Geometry check sheet. Reference: the model listing, model coordinates, mm. Round coordinates to 2 decimals unless told otherwise and drop trailing zeros. Loops run counter-clockwise (first coordinate to the right, second up) from the corner with the lowest first, then second, coordinate; pieces in that order, holes last. Notation, with made-up numbers: (-38, 54) - (-31, 54) arc R27 ccw to (-31, 93) - close; hole circle Ø3 at (50.5, 62). An arc over 180 degrees is marked (long way). Answer in a Markdown table with one row per item. Add a question column.
Autodesk Inventor part; units mm, degrees
ref_plane "YZ Plane" through (0, 0, 0) normal (1, 0, 0) x (0, 1, 0)
ref_plane "XZ Plane" through (0, 0, 0) normal (0, 1, 0) x (-1, 0, 0)
ref_plane "XY Plane" through (0, 0, 0) normal (0, 0, 1) x (1, 0, 0)
sketch "Sketch1" plane through (0, 0, 0) normal (0, 0, 1) x (1, 0, 0)
  line L0 (21.0847, 68.8136) -> (-66.9153, 68.8136)
  line L1 (-70.9153, 72.8136) -> (-70.9153, 145.8136)
  line L2 (-66.9153, 149.8136) -> (21.0847, 149.8136)
  line L3 (25.0847, 145.8136) -> (25.0847, 72.8136)
  line L4 (4.925, 0) -> (4.925, 205.34)
  line L5 (-25.075, 0) -> (-25.075, 205.34)
  arc A0 (-66.9153, 149.8136) -> (-70.9153, 145.8136) centre (-66.9153, 145.8136) ccw
  arc A1 (25.0847, 145.8136) -> (21.0847, 149.8136) centre (21.0847, 145.8136) ccw
  arc A2 (21.0847, 68.8136) -> (25.0847, 72.8136) centre (21.0847, 72.8136) ccw
  arc A3 (-70.9153, 72.8136) -> (-66.9153, 68.8136) centre (-66.9153, 72.8136) ccw
  point P0 (0, 0)
  dimension "d0" = 96
  dimension "d1" = 81
  dimension "d2" = 4
extrude "Extrusion1" add sketch "Sketch1" along normal blind 4.7
sketch "Sketch2" plane through (0, 0, 4.7) normal (0, 0, 1) x (1, 0, 0)
  line L0 (21.0847, 149.8136) -> (-66.9153, 149.8136)
  arc A0 (-66.9153, 149.8136) -> (-70.9153, 145.8136) centre (-66.9153, 145.8136) ccw
  line L1 (-70.9153, 145.8136) -> (-70.9153, 72.8136)
  arc A1 (-70.9153, 72.8136) -> (-66.9153, 68.8136) centre (-66.9153, 72.8136) ccw
  line L2 (-66.9153, 68.8136) -> (21.0847, 68.8136)
  arc A2 (21.0847, 68.8136) -> (25.0847, 72.8136) centre (21.0847, 72.8136) ccw
  line L3 (25.0847, 72.8136) -> (25.0847, 145.8136)
  arc A3 (25.0847, 145.8136) -> (21.0847, 149.8136) centre (21.0847, 145.8136) ccw
  circle A4 centre (-50.9153, 109.3136) radius 7.448
  point P0 (0, 0)
  dimension "d5" = 20
extrude "Extrusion2" cut sketch "Sketch2" against normal through all contours A4
properties part number "Neje_Base_slide_x"
Q1. Cross-section at B-B, the plane z = 2.65. Enter the section's corners in (x, y), plus the area to 3 significant figures.
Q2. Release check for a two-part mould opening along X. For faces 1 (the cylindrical face through (-69.71, 69.95, 2.32)), 2 (the cylindrical face through (-47.479, 102.706, 2.383)), 3 (the flat face through (-24, 110, 0)), 4 (the cylindrical face through (23.944, 70.016, 2.317)) record: +X half, -X half, draft (parallel to the pull), parting line (faces both ways), or undercut.
Q3. Scan lines: line 1 (X direction, y = 106, z = 2.3); line 2 (X direction, y = 115, z = 1); line 3 (Y direction, x = -54.5, z = 1.9) (3 decimals). Record each from-to range of solid material in increasing order. Write a range as from..to.
Q4. Depth check by flat-ended pin: P1, Ø12, axis at x = -50.92, y = 109.31, coming from the -Z side. Enter the tip coordinate at first touch or a pass-through.
Q5. Cross-section at A-A, the plane x = -51.5. Enter the section's corners in (y, z), plus the area to 3 significant figures.
Check sheet entries:
| question | item | result |
|---|---|---|
| 1 | outline | (-70.92, 72.81) arc R4 ccw to (-66.92, 68.81) - (21.08, 68.81) arc R4 ccw to (25.08, 72.81) - (25.08, 145.81) arc R4 ccw to (21.08, 149.81) - (-66.92, 149.81) arc R4 ccw to (-70.92, 145.81) - close; hole circle Ø14.9 at (-50.92, 109.31) |
| 1 | area | 7,590 mm² |
| 2 | face 1 | -X half |
| 2 | face 2 | undercut |
| 2 | face 3 | draft |
| 2 | face 4 | +X half |
| 3 | line 1 | -70.92..-57.59, -44.25..25.08 |
| 3 | line 2 | -70.92..-55.73, -46.11..25.08 |
| 3 | line 3 | 68.814..102.785, 115.842..149.814 |
| 4 | P1 | through |
| 5 | outline | (68.81, 0) - (101.89, 0) - (101.89, 4.7) - (68.81, 4.7) - close; (116.74, 0) - (149.81, 0) - (149.81, 4.7) - (116.74, 4.7) - close |
| 5 | area | 311 mm² |
